```python
from build123d import *

# Parameters (mm, degrees)
F0_R         = 11
F1_DEPTH     = 6.35
F2_SIZE      = 3.17499
F3_T2_ANGLE  = 199.5715846066
F3_T4_ANGLE  = 199.5715846066
F3_T6_ANGLE  = 199.5715846066
F3_T8_ANGLE  = 199.5715846066
F3_T10_ANGLE = 199.5715846066
F3_T12_ANGLE = 199.5715846066
F3_T14_ANGLE = 199.5715846066
F3_T16_ANGLE = 199.5715846066
F3_T18_ANGLE = 199.5715846066
F3_T20_ANGLE = 199.5715846066


# Not quite as in the source:
# - a fillet or chamfer that OpenCascade refuses, or shapes differently, is made with other operations: its cross-section is extruded or revolved along the edge and cut away or added
# - a fillet or chamfer is up to 0.001 mm smaller than in the source, because OpenCascade refuses the exact size


with BuildPart() as f1:
    # F0 (on Front) → F1 (new body)
    with BuildSketch(Plane.XZ):
        with BuildLine():
            Line((11.5903794876, 19.7357752055), (6.395639386, 25.8985348046))
            Line((6.395639386, 25.8985348046), (-1.0707562618, 22.8624408289))
            ThreePointArc((-1.0707562618, 22.8624408289), (-0.6511189694, 21.4544603732), (-0.5094848211, 19.9921183513))
            ThreePointArc((-0.5094848211, 19.9921183513), (-6.6671427992, 12.5137524996), (-15.1882133804, 17.1217958736))
            Line((-15.1882133804, 17.1217958736), (-22.6546090282, 14.085701898))
            Line((-22.6546090282, 14.085701898), (-22.0743552105, 6.0465330289))
            ThreePointArc((-22.0743552105, 6.0465330289), (-16.3352014079, 4.025037517), (-13.9057833978, -1.5536951891))
            ThreePointArc((-13.9057833978, -1.5536951891), (-15.9470506916, -6.744277179), (-20.977211585, -9.1539234072))
            Line((-20.977211585, -9.1539234072), (-20.3969577673, -17.1930922762))
            Line((-20.3969577673, -17.1930922762), (-12.5719455381, -19.125477903))
            ThreePointArc((-12.5719455381, -19.125477903), (-4.2540087238, -13.3881176755), (2.4458190468, -20.9523547863))
            ThreePointArc((2.4458190468, -20.9523547863), (2.3900561576, -21.8725270157), (2.2235836317, -22.7792316697))
            Line((2.2235836317, -22.7792316697), (10.0485958609, -24.7116172964))
            Line((10.0485958609, -24.7116172964), (14.3044655632, -17.866728424))
            ThreePointArc((14.3044655632, -17.866728424), (11.8568074939, -7.3720740717), (22.3514618462, -4.9244160023))
            Line((22.3514618462, -4.9244160023), (26.6073315486, 1.9204728701))
            Line((26.6073315486, 1.9204728701), (21.412591447, 8.0832324691))
            ThreePointArc((21.412591447, 8.0832324691), (10.6752140991, 8.9983978576), (11.5903794876, 19.7357752055))
        make_face()
        Circle(F0_R, mode=Mode.SUBTRACT)
    extrude(amount=F1_DEPTH)

    # F2 (size 3.175 in the source; OpenCascade refuses exactly that, so slightly less here)
    f2_edges = [f1.edges().sort_by_distance(p)[0] for p in [
        (24.479397, -6.35, -1.501972),
        (24.009961, -6.35, 5.001853),
        (8.993009, -6.35, 22.817155),
        (2.662442, -6.35, 24.380488),
        (-18.921411, -6.35, 15.603749),
        (-22.364482, -6.35, 10.066117),
        (-20.687085, -6.35, -13.173508),
        (-16.484452, -6.35, -18.159285),
        (24.009961, 0, 5.001853),
        (24.479397, 0, -1.501972),
        (8.993009, 0, 22.817155),
        (2.662442, 0, 24.380488),
        (-18.921411, 0, 15.603749),
        (-22.364482, 0, 10.066117),
        (-20.687085, 0, -13.173508),
        (-16.484452, 0, -18.159285),
        (6.13609, 0, -23.745424),
        (12.176531, 0, -21.289173),
        (12.176531, -6.35, -21.289173),
        (6.13609, -6.35, -23.745424),
    ]]
    chamfer(f2_edges, length=F2_SIZE)

    # F3: chamfer of 1.778 on 10 edges, made by hand

    # F3_s1 → F3_t2 (revolve, cut)
    with BuildSketch(Plane(origin=(19.7071717725, 0, -7.9965849701), x_dir=(0, 1, 0), z_dir=(0.9266214967, 0, -0.3759954812))):
        Polygon((-1.778, -11.2881506475), (0, -13.0661506475), (0, -11.2881506475), align=None)
    revolve(axis=Axis((18.3279637047, 0, -11.3955722132), (0, 1, 0)), revolution_arc=F3_T2_ANGLE, mode=Mode.SUBTRACT)

    # F3_s3 → F3_t4 (revolve, cut)
    with BuildSketch(Plane(origin=(19.7071717725, 0, -7.9965849701), x_dir=(0, 1, 0), z_dir=(0.9266214967, 0, -0.3759954812))):
        Polygon((-4.572, -11.2881506475), (-6.35, -13.0661506475), (-6.35, -11.2881506475), align=None)
    revolve(axis=Axis((18.3279637047, -6.35, -11.3955722132), (0, 1, 0)), revolution_arc=F3_T4_ANGLE, mode=Mode.SUBTRACT)

    # F3_s5 → F3_t6 (revolve, cut)
    with BuildSketch(Plane(origin=(-8.534063628, 0, -19.4804452837), x_dir=(0, 1, 0), z_dir=(-0.4012674626, 0, -0.915960929))):
        Polygon((-6.35, 13.0661506475), (-4.572, 11.2881506475), (-6.35, 11.2881506475), align=None)
    revolve(axis=Axis((-5.1741809532, -6.35, -20.9523547863), (0, -1, 0)), revolution_arc=F3_T6_ANGLE, mode=Mode.SUBTRACT)

    # F3_s7 → F3_t8 (revolve, cut)
    with BuildSketch(Plane(origin=(-1.5153532552, 0, -21.2137147847), x_dir=(0, 1, 0), z_dir=(-0.0712511627, 0, -0.9974584061))):
        Polygon((0, -13.0661506475), (-1.778, -11.2881506475), (0, -11.2881506475), align=None)
    revolve(axis=Axis((-5.1741809532, 0, -20.9523547863), (0, 1, 0)), revolution_arc=F3_T8_ANGLE, mode=Mode.SUBTRACT)

    # F3_s9 → F3_t10 (revolve, cut)
    with BuildSketch(Plane(origin=(-21.1641751195, 0, 2.0965881732), x_dir=(0, 1, 0), z_dir=(-0.9951290754, 0, 0.0985805418))):
        Polygon((-6.35, 13.0661506475), (-4.572, 11.2881506475), (-6.35, 11.2881506475), align=None)
    revolve(axis=Axis((-21.5257833978, -6.35, -1.5536951891), (0, -1, 0)), revolution_arc=F3_T10_ANGLE, mode=Mode.SUBTRACT)

    # F3_s11 → F3_t12 (revolve, cut)
    with BuildSketch(Plane(origin=(-20.6437115892, 0, -5.1142117945), x_dir=(0, 1, 0), z_dir=(-0.9706571369, 0, -0.2404677161))):
        Polygon((0, -13.0661506475), (-1.778, -11.2881506475), (0, -11.2881506475), align=None)
    revolve(axis=Axis((-21.5257833978, 0, -1.5536951891), (0, 1, 0)), revolution_arc=F3_T12_ANGLE, mode=Mode.SUBTRACT)

    # F3_s13 → F3_t14 (revolve, cut)
    with BuildSketch(Plane(origin=(-4.5461159397, 0, 20.7762080351), x_dir=(0, 1, 0), z_dir=(-0.2137561292, 0, 0.9768870545))):
        Polygon((-6.35, 13.0661506475), (-4.572, 11.2881506475), (-6.35, 11.2881506475), align=None)
    revolve(axis=Axis((-8.1294848211, -6.35, 19.9921183513), (0, -1, 0)), revolution_arc=F3_T14_ANGLE, mode=Mode.SUBTRACT)

    # F3_s15 → F3_t16 (revolve, cut)
    with BuildSketch(Plane(origin=(-11.2431621609, 0, 18.0529580701), x_dir=(0, 1, 0), z_dir=(-0.5286479394, 0, 0.8488411843))):
        Polygon((0, -13.0661506475), (-1.778, -11.2881506475), (0, -11.2881506475), align=None)
    revolve(axis=Axis((-8.1294848211, 0, 19.9921183513), (0, 1, 0)), revolution_arc=F3_T16_ANGLE, mode=Mode.SUBTRACT)

    # F3_s17 → F3_t18 (revolve, cut)
    with BuildSketch(Plane(origin=(13.6950552327, 0, 16.2715534792), x_dir=(0, 1, 0), z_dir=(0.6439347423, 0, 0.7650804191))):
        Polygon((-6.35, -13.0661506475), (-4.572, -11.2881506475), (-6.35, -11.2881506475), align=None)
    revolve(axis=Axis((16.5014854673, -6.35, 13.9095038373), (0, 1, 0)), revolution_arc=F3_T18_ANGLE, mode=Mode.SUBTRACT)

    # F3_s19 → F3_t20 (revolve, cut)
    with BuildSketch(Plane(origin=(13.6950552327, 0, 16.2715534792), x_dir=(0, 1, 0), z_dir=(0.6439347423, 0, 0.7650804191))):
        Polygon((0, -13.0661506475), (-1.778, -11.2881506475), (0, -11.2881506475), align=None)
    revolve(axis=Axis((16.5014854673, 0, 13.9095038373), (0, 1, 0)), revolution_arc=F3_T20_ANGLE, mode=Mode.SUBTRACT)


solid = f1.part
```
Geometry check sheet. Reference: the model listing, model coordinates, mm. Round coordinates to 2 decimals unless told otherwise and drop trailing zeros. Order: outer loops, then holes, each group sorted by start corner. A loop starts at its lowest first (then second) coordinate and runs counter-clockwise, first axis right, second up. Notation, with made-up numbers: (72, 89.5) -> (101, 89.5) arc R22 ccw to (101, 104.5) -> close; hole circle Ø11 at (21, -7.5). An arc over 180 degrees is marked (long way). Return JSON: item names as keys, results as strings. Group by question number.
Q1. Material ranges on probe 1 along Z at (x, y) = (-1, -0.25); probe 2 along X at (y, z) = (-3.5, 1.5); probe 3 along X at (y, z) = (-2, -16), recorded low to high. Write a range as from..to.
Q2. Section check A-A, the plane y = -2.5. Record the boundary of the cut face in (x, z).
Q3. Gauge pin test, flat ends, axial feed: pin 1 (2 mm diameter, centred on x = -6, y = -1, fed in from +Z); pin 2 (3 mm diameter, centred on y = -1, z = 1, fed in from -X); pin 3 (1 mm diameter, centred on y = -1, z = -16, fed in from +X). Record the tip position at first contact, or that the pin passes through.
Q4. Release check for a two-part mould opening along Z. For faces 1 (the cylindrical face through (-2.38, -3.13, -10.74)), 2 (the flat face through (22.774, -4.785, 3.97)), 3 (the flat face through (23, -4.8, -0.8)) record: released by +Z, released by -Z, zero draft, split by the parting line, or undercut.
Numbers:
{
 "1": {"probe 1": "-12.81..-10.95, 10.95..14.26", "probe 2": "-14.54..-10.9, 10.9..25.96", "probe 3": "-19.31..-10.97, 0.62..12.26"},
 "2": {"outline": "(-21.95, 13.65) -> (-21.4, 6.07) arc R7.62 cw to (-20.31, -9.08) -> (-19.76, -16.66) -> (-12.38, -18.48) arc R7.62 cw to (2.36, -22.12) -> (9.73, -23.94) -> (13.75, -17.48) arc R7.62 cw to (21.76, -4.59) -> (25.78, 1.86) -> (20.88, 7.67) arc R7.62 cw to (11.09, 19.28) -> (6.2, 25.09) -> (-0.84, 22.23) arc R7.62 cw to (-14.91, 16.51) -> close; hole circle Ø22 at (0, 0)"},
 "3": {"pin 1": "z = 12.89", "pin 2": "x = -14.94", "pin 3": "x = 12.01"},
 "4": {"face 1": "undercut", "face 2": "released by +Z", "face 3": "released by -Z"}
}
